Autodesk Inventor part; units mm, degrees
ref_plane "YZ Plane" through (0, 0, 0) normal (1, 0, 0) x (0, 1, 0)
ref_plane "XZ Plane" through (0, 0, 0) normal (0, 1, 0) x (-1, 0, 0)
ref_plane "XY Plane" through (0, 0, 0) normal (0, 0, 1) x (1, 0, 0)
sketch "Sketch1" plane through (0, 0, 0) normal (0, 0, 1) x (1, 0, 0)
  line L0 (-0.8746, 32.779) -> (-0.8746, -34.5944)
  line L1 (22.6254, 4.1775) -> (53.6254, 4.1775)
  line L2 (53.6254, 4.1775) -> (53.6254, -20.8225)
  line L3 (53.6254, -20.8225) -> (22.6254, -20.8225)
  line L4 (22.6254, -20.8225) -> (22.6254, 4.1775)
  line L5 (38.1254, 4.1775) -> (38.1254, -20.8225)
  line L6 (38.1254, 15.3436) -> (43.2254, 15.3436)
  line L7 (43.2254, 15.3436) -> (43.2254, -23.8453)
  line L8 (43.2254, -23.8453) -> (38.1254, -23.8453)
  line L9 (38.1254, -23.8453) -> (38.1254, 15.3436)
  line L10 (22.6254, -15.8225) -> (17.6254, -15.8225)
  line L11 (17.6254, -15.8225) -> (17.6254, -20.8225)
  line L12 (17.6254, -20.8225) -> (22.6254, -20.8225)
  line L13 (22.6254, -20.8225) -> (22.6254, -15.8225)
  point P0 (0, 0)
  dimension "d0" = 47
  dimension "d1" = 25
  dimension "d3" = 39
  dimension "d5" = 10.2
  dimension "d7" = 5
  dimension "d8" = 5
revolve "Revolution1" add sketch "Sketch1" angle 360 about axis through (-0.8746, 32.779, 0) along (0, -1, 0) contours L1 L5 L3 L4 | L1 L7 L3 L5 | L1 L2 L3 L7
revolve "Revolution2" cut sketch "Sketch1" angle 360 about axis through (38.1254, -23.8453, 0) along (0, 1, 0) contours L9 L6 L7 L1 | L1 L7 L3 L5 | L3 L7 L8 L9
revolve "Revolution3" add sketch "Sketch1" angle 360 about axis through (-0.8746, 32.779, 0) along (0, -1, 0) contours L4 L12 L11 L10
pattern_circular "Circular Pattern1" count 6 over 360 about axis through (-0.8746, -8.3225, 0) along (0, -1, 0) of "Revolution2"
sketch "Sketch2" plane through (-0.8746, -20.8225, 0) normal (0, -1, 0) x (1, 0, 0)
  circle A0 centre (-0.347, 62) radius 15
  circle A1 centre (19.5, -33.775) radius 5.1
  circle A2 centre (-19.5, -33.775) radius 5.1
  circle A3 centre (-39, 0) radius 5.1
  circle A4 centre (-19.5, 33.775) radius 5.1
  circle A5 centre (19.5, 33.775) radius 5.1
  circle A6 centre (0, 0) radius 18.5
  circle A7 centre (39, 0) radius 5.1
  circle A8 centre (0, 0) radius 54.5
  point P0 (0.8746, 0)
  dimension "d13" = 62
  dimension "d14" = 30
extrude "Extrusion1" cut sketch "Sketch2" against normal through all contours A0 A8 | A8 A0 picked at (-0.731, 61.8812) picked at (-0.2905, 51.8983)
pattern_circular "Circular Pattern2" count 6 over 360 about axis through (-0.8746, -8.3225, 0) along (0, -1, 0) of "Extrusion1"
properties part number "HELP_6204BEARING_CASE_A"
Build history of the part. All positions in model axes, mm. A direction names the side the tool comes from. Round coordinates to 2 decimals unless told otherwise and drop trailing zeros. Write each loop counter-clockwise with the first axis right and the second up, starting at its lowest first coordinate (ties: lowest second). Pieces come first, ordered by that corner, then holes. Notation, with made-up numbers: (62.25, 17.5) -> (92.25, 17.5) arc R32 ccw to (92.25, 53.5) -> close; hole circle Ø9 at (-35, -15.5). An arc over 180 degrees is marked (long way). Put each result on its own line as item: value.
Item 1: Slice it at B-B, the plane y = -9.25. Give the cut face in (x, z) (3 decimals), plus the area to 3 significant figures.
Here are the results:
outline: (-53.035, 15.797) arc R54.5 ccw to (-52.855, -16.38) arc R15 cw to (-40.635, -37.274) arc R54.5 ccw to (-12.679, -53.206) arc R15 cw to (11.525, -53.071) arc R54.5 ccw to (39.301, -36.826) arc R15 cw to (51.286, -15.797) arc R54.5 ccw to (51.106, 16.38) arc R15 cw to (38.886, 37.274) arc R54.5 ccw to (10.93, 53.206) arc R15 cw to (-13.274, 53.071) arc R54.5 ccw to (-41.05, 36.826) arc R15 cw to start; hole circle Ø10.2 at (-39.875, 0); hole circle Ø10.2 at (-20.375, -33.775); hole circle Ø10.2 at (-20.375, 33.775); hole circle Ø47 at (-0.875, 0); hole circle Ø10.2 at (18.625, -33.775); hole circle Ø10.2 at (18.625, 33.775); hole circle Ø10.2 at (38.125, 0)
area: 6,350 mm^2
Item 2: Slice it at C-C, the plane x = 31. Give the cut face in (y, z), plus the area to 3 significant figures.
Here are the results:
outline: (-20.82, -44.21) -> (4.18, -44.21) -> (4.18, 44.21) -> (-20.82, 44.21) -> close
area: 2,210 mm^2
Item 3: Wall check: probe 1 along Z at (x, y) = (16, -3); probe 2 along Z at (x, y) = (-16, -7.5); probe 3 along Z at (x, y) = (-0.5, -8.75). Give the ranges that are in metal, low to high. Write a range as from..to.
Here are the results:
probe 1: z = -51.82..-38.15, -29.4..-16.36, 16.36..29.4, 38.15..51.82
probe 2: z = -52.36..-36.4, -31.15..-17.99, 17.99..31.15, 36.4..52.36
probe 3: z = -47..-23.5, 23.5..47.02
Item 4: Tool access for faces 1 (the face through (-18.2, -5.68, -15.88)), 2 (the face through (40.06, -8.5, -23.1)): list every direction of +Z, -Z, +X, -X, +Y, -Y with a clear straight run to the whole face (end or side of a thin tool).
Here are the results:
face 1: +Y
face 2: +X, +Y, -Y
Item 5: Flat gauge pins, fed straight in: P1, Ø13.5, axis at x = -20.37, z = -33.77, coming from the +Y side; P2, Ø4, axis at y = -18, z = 20.5, coming from the +X side; P3, Ø4, axis at x = 8, y = -8, coming from the -Z side (3 decimals); P4, Ø12, axis at y = -12, z = 21.5, coming from the -X side. Where does each tip first touch, or does it go through?
Here are the results:
P1: stops at y = 4.18
P2: stops at x = 44.83
P3: stops at z = -51.315
P4: stops at x = -53.12
Item 6: Slice it at A-A, the plane z = -8.5. Give the cut face in (x, y), plus the area to 3 significant figures.
Here are the results:
outline: (-54.71, -20.82) -> (-17.31, -20.82) -> (-17.31, -15.82) -> (-22.78, -15.82) -> (-22.78, 4.18) -> (-54.71, 4.18) -> close; (15.56, -20.82) -> (52.96, -20.82) -> (52.96, 4.18) -> (21.03, 4.18) -> (21.03, -15.82) -> (15.56, -15.82) -> close
area: 1,650 mm^2
Item 7: Two-plate mould, pull along Z, no slides. Class faces 3 (the face through (53.625, -8.498, 0.076)), 4 (the face through (-41.81, -8.5, 23.1)), 5 (the face through (-26, 4.178, 1)): pulls with the +Z half, pulls with the -Z half, needs draft (parallel to the pull), parting line crosses it, or undercut.
Here are the results:
face 3: parting line crosses it
face 4: undercut
face 5: needs draft
